The model under review builds one solid part; all positions refer to its coordinate system, in mm. Face numbers are marked on the shaded views. A direction names the side the tool comes from. Give positions to 0.01 mm unless a question says otherwise; leave off trailing zeros. Write each loop counter-clockwise with the first axis right and the second up, starting at its lowest first coordinate (ties: lowest second). Pieces come first, ordered by that corner, then holes. Notation, with made-up numbers: M 71,2 L 91,2 A23 cw 91,20 Z; hole C -33,87 d7. An arc over 180 degrees is marked long. Write each question's results on one line, items separated by ' | '. Start each with the question number.
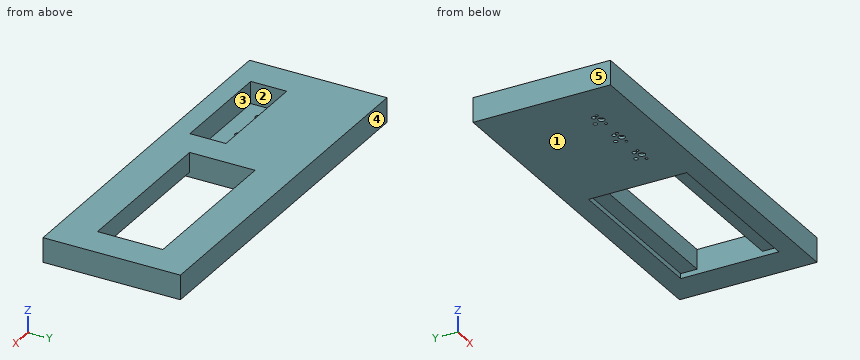
Autodesk Fusion 360 part; units mm, degrees
sketch "Sketch1" plane through (0, 0, 0) normal (0, 0, 1) x (1, 0, 0)
  line L0 (112, 42) -> (-112, 42)
  line L1 (-112, 42) -> (-112, -42)
  line L2 (-112, -42) -> (112, -42)
  line L3 (112, -42) -> (112, 42)
  line L4 (112, 42) -> (-112, -42) construction
  line L5 (-112, 42) -> (112, -42) construction
  line L6 (-8, 30) -> (92, 30)
  line L7 (92, 30) -> (92, -30)
  line L8 (92, -30) -> (-8, -30)
  line L9 (-8, -30) -> (-8, 30)
  line L10 (-8, 30) -> (92, -30) construction
  line L11 (92, 30) -> (-8, -30) construction
  line L12 (92, 20) -> (-8, 20)
  line L13 (-8, 20) -> (-8, -20)
  line L14 (-8, -20) -> (92, -20)
  line L15 (92, -20) -> (92, 20)
  line L16 (92, 20) -> (-8, -20) construction
  line L17 (-8, 20) -> (92, -20) construction
  line L18 (92, 42) -> (92, -42) construction
  line L19 (-81, -19) -> (-78.46, -19) construction
  line L20 (-81, -13.92) -> (-81, -19) construction
  circle A0 centre (-75.92, -19) radius 0.85
  line L21 (-81, -16.46) -> (-81, -19) construction
  line L22 (-84.81, -19) -> (-84.81, -16.46) construction
  line L23 (-78.46, -13.92) -> (-81, -13.92) construction
  circle A1 centre (-78.46, -13.92) radius 1.25
  circle A2 centre (-86.08, -19) radius 0.85
  circle A3 centre (-81, -19) radius 2
  circle A4 centre (-84.81, -16.46) radius 1.25
  line L24 (-78.46, -19) -> (-78.46, -13.92) construction
  line L25 (-81, -19) -> (-75.92, -19) construction
  line L26 (-81, -19) -> (-84.81, -19) construction
  line L27 (-84.81, -16.46) -> (-81, -16.46) construction
  line L28 (-70, -8) -> (-92, -8)
  line L29 (-92, -8) -> (-92, -30)
  line L30 (-92, -30) -> (-70, -30)
  line L31 (-70, -30) -> (-70, -8) construction
  line L32 (-70, -8) -> (-92, -30) construction
  line L33 (-92, -8) -> (-70, -30) construction
  circle A5 centre (-53.92, -19) radius 0.85
  line L34 (-56.46, -19) -> (-56.46, -13.92) construction
  circle A6 centre (-64.08, -19) radius 0.85
  circle A7 centre (-62.81, -16.46) radius 1.25
  line L35 (-59, -16.46) -> (-59, -19) construction
  line L36 (-48, -30) -> (-48, -8) construction
  line L37 (-59, -19) -> (-53.92, -19) construction
  line L38 (-70, -8) -> (-48, -30) construction
  line L39 (-56.46, -13.92) -> (-59, -13.92) construction
  line L40 (-70, -8) -> (-70, -30) construction
  circle A8 centre (-56.46, -13.92) radius 1.25
  circle A9 centre (-59, -19) radius 2
  line L41 (-59, -19) -> (-56.46, -19) construction
  line L42 (-48, -8) -> (-70, -8)
  line L43 (-59, -13.92) -> (-59, -19) construction
  line L44 (-48, -8) -> (-70, -30) construction
  line L45 (-70, -30) -> (-48, -30)
  line L46 (-62.81, -19) -> (-62.81, -16.46) construction
  line L47 (-59, -19) -> (-62.81, -19) construction
  line L48 (-62.81, -16.46) -> (-59, -16.46) construction
  circle A10 centre (-31.92, -19) radius 0.85
  line L49 (-34.46, -19) -> (-34.46, -13.92) construction
  circle A11 centre (-42.08, -19) radius 0.85
  circle A12 centre (-40.81, -16.46) radius 1.25
  line L50 (-37, -16.46) -> (-37, -19) construction
  line L51 (-26, -30) -> (-26, -8)
  line L52 (-37, -19) -> (-31.92, -19) construction
  line L53 (-48, -8) -> (-26, -30) construction
  line L54 (-34.46, -13.92) -> (-37, -13.92) construction
  line L55 (-48, -8) -> (-48, -30) construction
  circle A13 centre (-34.46, -13.92) radius 1.25
  circle A14 centre (-37, -19) radius 2
  line L56 (-37, -19) -> (-34.46, -19) construction
  line L57 (-26, -8) -> (-48, -8)
  line L58 (-37, -13.92) -> (-37, -19) construction
  line L59 (-26, -8) -> (-48, -30) construction
  line L60 (-48, -30) -> (-26, -30)
  line L61 (-40.81, -19) -> (-40.81, -16.46) construction
  line L62 (-37, -19) -> (-40.81, -19) construction
  line L63 (-40.81, -16.46) -> (-37, -16.46) construction
  line L64 (-92, -30) -> (-112, -30) construction
  line L65 (-112, -30) -> (-112, -42) construction
  line L66 (-112, -42) -> (-92, -42) construction
  line L67 (-92, -42) -> (-92, -30) construction
  point P0 (42, 0)
  point P1 (42, 0)
  point P2 (-81, -19)
  point P3 (-81, -19)
  point P4 (-81, -19)
  point P5 (-59, -19)
  point P6 (-59, -19)
  point P7 (-59, -19)
  point P8 (-37, -19)
  point P9 (-37, -19)
  point P10 (-37, -19)
  dimension "d1" = 224
  dimension "d2" = 84
  dimension "d3" = 100
  dimension "d4" = 60
  dimension "d5" = 100
  dimension "d6" = 40
  dimension "d7" = 4
  dimension "d8" = 5.08
  dimension "d9" = 1.7
  dimension "d10" = 2.54
  dimension "d11" = 5.08
  dimension "d12" = 2.5
  dimension "d13" = 3.81
  dimension "d14" = 2.54
  dimension "d15" = 2.5
  dimension "d16" = 22
  dimension "d17" = 22
  dimension "d20" = 44
  dimension "d21" = 0
  dimension "d22" = 20
  dimension "d23" = 12
  dimension "d24" = 20
extrude "Extrude1" add sketch "Sketch1" along normal blind 15 contours L0 L1 L2 L3
extrude "Extrude2" add sketch "Sketch1" along normal blind 1.5 contours L28 L29 L30 L42 L45 L51 L57 L60
extrude "Extrude3" add sketch "Sketch1" against normal blind 12 from surface at 15 contours L6 L7 L9 L12 | L7 L8 L9 L14
(1) Draft analysis for pull direction X (two halves, no side actions). For the marked faces 3, 4 and 5, state which applies: pulls with the +X half, pulls with the -X half, needs draft (parallel to the pull), parting line crosses it, or undercut.
(2) Add section C-C (x = -70.5). State the section outline as (y, z) points.
(3) Add section A-A (x = 24). State the section outline as (y, z) points.
(4) Machinability: for the marked faces 1 and 2, which of the approach directions +Z, -Z, +X, -X, +Y, -Y give a long, thin tool a straight path to every point of the face, cutting with its end or side? Answer none if there is none.
(5) Wall thickness on L1, parallel to X at y = -16, z = 7.5; L2, parallel to Y at x = -56.46, z = 0.4; L3, parallel to X at y = 14.5, z = 8.25: over which ranges is each line inside the solid? List them lowest first.
(6) Add section B-B (z = 11.75). State the section outline as (x, y) points, then the cut area to 3 significant figures.
(7) Clearance check with flat-ended pins moving along their axes: P1, Ø2, axis at x = -75.92, y = -19, coming from the +Z side; P2, Ø3, axis at x = 53, y = 22.5, coming from the -Z side; P3, Ø2, axis at x = -56.46, y = -13.92, coming from the -Z side. State where each tip first meets the part, or that it passes through.
(8) Add section D-D (y = -24). State the section outline as (x, z) points, then the cut area to 3 significant figures.
Calculated:
1) face 3: undercut | face 4: needs draft | face 5: pulls with the -X half
2) outline: M -42,0 L 42,0 L 42,15 L -8,15 L -8,1.5 L -30,1.5 L -30,15 L -42,15 Z
3) outline: M -42,0 L -30,0 L -30,3 L -20,3 L -20,15 L -42,15 Z; M 20,3 L 30,3 L 30,0 L 42,0 L 42,15 L 20,15 Z
4) face 1: -Z, +X, -X, +Y, -Y | face 2: +Z
5) L1: x = -112 to -92, -26 to -8, 92 to 112 | L2: y = -42 to -15.17, -12.67 to 42 | L3: x = -112 to -8, 92 to 112
6) outline: M -112,-42 L 112,-42 L 112,42 L -112,42 Z; hole M -92,-30 L -26,-30 L -26,-8 L -92,-8 Z; hole M -8,-20 L 92,-20 L 92,20 L -8,20 Z | area: 13,400 mm²
7) P1: stops at z = 1.5 | P2: stops at z = 3 | P3: passes through
8) outline: M -112,0 L -8,0 L -8,3 L 92,3 L 92,0 L 112,0 L 112,15 L -26,15 L -26,1.5 L -92,1.5 L -92,15 L -112,15 Z | area: 2,170 mm²
